Read the model definition and answer for the solid it produces. Units are mm, in the model's axes. A direction names the side the tool comes from. Give positions to 0.01 mm unless a question says otherwise; leave off trailing zeros. Write each loop counter-clockwise with the first axis right and the second up, starting at its lowest first coordinate (ties: lowest second). Pieces come first, ordered by that corner, then holes.
```python
from build123d import *

# Parameters (mm, degrees)
SKETCH_1_W          = 16.6
SKETCH_1_H          = 22
SKETCH_1_R          = 4.1
SKETCH_1_R_2        = 1.25
EXTRUDE_1_DEPTH     = 3.5
SKETCH_1_3_R        = 4.1
SKETCH_1_3_R_2      = 2.8
EXTRUDE_2_DEPTH     = 1
FILLET_1_R          = 10
FILLET_2_R          = 5
SKETCH_2_R          = 1
CUT_EXTRUDE_1_DEPTH = 6
SKETCH_2_3_R        = 1.5
EXTRUDE_3_DEPTH     = 1.6


with BuildPart() as part:
    # Sketch 1 → Extrude 1 (new body)
    with BuildSketch(Plane.XY):
        with Locations((-3.7, 1)):
            Rectangle(SKETCH_1_W, SKETCH_1_H)
        Circle(SKETCH_1_R, mode=Mode.SUBTRACT)
        with Locations((0, 8)):
            Circle(SKETCH_1_R_2, mode=Mode.SUBTRACT)
        with Locations((-8, 0)):
            Circle(SKETCH_1_R_2, mode=Mode.SUBTRACT)
    extrude(amount=EXTRUDE_1_DEPTH)

    # Sketch 1_3 → Extrude 2 (add)
    with BuildSketch(Plane.XY):
        Circle(SKETCH_1_3_R)
        Circle(SKETCH_1_3_R_2, mode=Mode.SUBTRACT)
    extrude(amount=EXTRUDE_2_DEPTH)

    # Fillet 1
    fillet_1_edges = [part.edges().sort_by_distance(p)[0] for p in [
        (-12, 12, 1.75),
    ]]
    fillet(fillet_1_edges, radius=FILLET_1_R)

    # Fillet 2
    fillet_2_edges = [part.edges().sort_by_distance(p)[0] for p in [
        (4.6, 12, 1.75),
    ]]
    fillet(fillet_2_edges, radius=FILLET_2_R)

    # Sketch 2 → Cut-Extrude 1 (cut)
    with BuildSketch(Plane.XZ.offset(10)):
        with Locations(Location((-4.5, 1.75, 0), (0, 0, 270))):
            Circle(SKETCH_2_R)
    extrude(amount=-CUT_EXTRUDE_1_DEPTH, mode=Mode.SUBTRACT)

    # Sketch 2_3 → Extrude 3 (add)
    with BuildSketch(Plane.XZ.offset(10)):
        with Locations(Location((-10.5, 1.75, 0), (0, 0, 180))):
            Circle(SKETCH_2_3_R)
    extrude(amount=EXTRUDE_3_DEPTH)


solid = part.part
```
Item 1: Find the intervals of material crossed by line 1 along X through (y, z) = (-3, 3); line 2 along Y through (x, z) = (0, 0.5); line 3 along Y through (x, z) = (0, 2.85), in increasing order.
Result set:
line 1: x = -12 to -2.79, 2.79 to 4.6
line 2: y = -10 to -2.8, 2.8 to 6.75, 9.25 to 11.98
line 3: y = -10 to -4.1, 4.1 to 6.75, 9.25 to 11.98
Item 2: Section C-C (x = 1) is taken. Write down the section's boundary in (y, z).
Result set:
outline: (-10, 0) - (-2.62, 0) - (-2.62, 1) - (-3.98, 1) - (-3.98, 3.5) - (-10, 3.5) - close; (2.62, 0) - (7.25, 0) - (7.25, 3.5) - (3.98, 3.5) - (3.98, 1) - (2.62, 1) - close; (8.75, 0) - (11.8, 0) - (11.8, 3.5) - (8.75, 3.5) - close
Item 3: Section D-D (z = 2.1) is taken. Write down the section's boundary in (x, y).
Result set:
outline: (-12, -10) - (-11.96, -10) - (-11.96, -11.6) - (-9.04, -11.6) - (-9.04, -10) - (-5.44, -10) - (-5.44, -4) - (-3.56, -4) - (-3.56, -10) - (4.6, -10) - (4.6, 7) arc R5 ccw to (-0.4, 12) - (-2, 12) arc R10 ccw to (-12, 2) - close; hole circle Ø2.5 at (-8, 0); hole circle Ø8.2 at (0, 0); hole circle Ø2.5 at (0, 8)
Item 4: Section A-A (x = -8) is taken. Write down the section's boundary in (y, z).
Result set:
outline: (-10, 0) - (-1.25, 0) - (-1.25, 3.5) - (-10, 3.5) - close; (1.25, 0) - (10, 0) - (10, 3.5) - (1.25, 3.5) - close
Item 5: Section B-B (y = 0) is taken. Write down the section's boundary in (x, z), and give its area (4 significant figures).
Result set:
outline: (-12, 0) - (-9.25, 0) - (-9.25, 3.5) - (-12, 3.5) - close; (-6.75, 0) - (-2.8, 0) - (-2.8, 1) - (-4.1, 1) - (-4.1, 3.5) - (-6.75, 3.5) - close; (2.8, 0) - (4.6, 0) - (4.6, 3.5) - (4.1, 3.5) - (4.1, 1) - (2.8, 1) - close
area: 23.25 mm2
Item 6: Which of the six approach directions +Z, -Z, +X, -X, +Y, -Y give full straight-line access (tool end or side, diameter ignored) to faces 4 (the cylindrical face through (-3.51, -7.04, 1.88)), 5 (the flat face through (1, -3, 1)), 6 (the flat face through (-1, 12, 2))?
Result set:
face 4: -Y
face 5: +Z
face 6: +Z, -Z, +X, -X, +Y
Item 7: Each of these flat-tipped pins is pushed along its axis until it touches: pin 1 Ø3.5 at (x, y) = (0, 0) entering from -Z; pin 2 Ø1.6 at (x, z) = (-4, 2) entering from -Y; pin 3 Ø1.8 at (x, z) = (-4.5, 1.75) entering from +Y. Where does it stop, or does it pass through?
Result set:
pin 1: passes through
pin 2: stops at y = -10
pin 3: stops at y = 11.87
Item 8: Determine the mould class of faces 1 (the flat face through (4.6, -2, 2)), 2 (the cylindrical face through (-0.534, 4.065, 2.232)), 3 (the flat face through (-6, 1, 3.5)) for opening direction X: pulls with the +X half, pulls with the -X half, needs draft (parallel to the pull), parting line crosses it, or undercut.
Result set:
face 1: pulls with the +X half
face 2: undercut
face 3: needs draft
